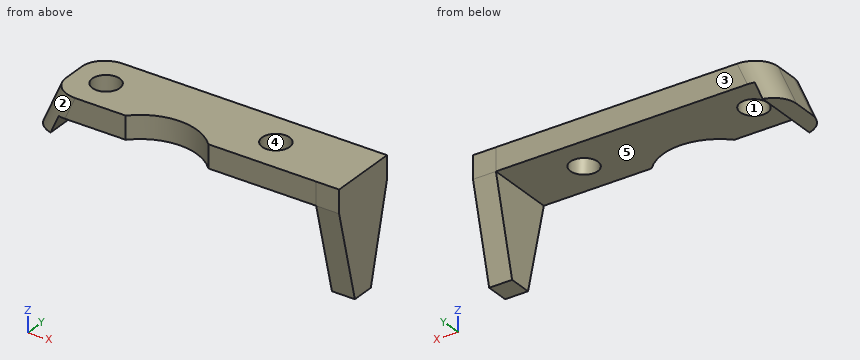
from build123d import *

# Parameters (mm, degrees)
F0_R     = 3
F1_DEPTH = 5
F2_W     = 15.0000307818
F2_H     = 5
F3_DEPTH = 5
F5_DEPTH = 15
F6_R     = 5


with BuildPart() as f1:
    # F0 (on Top) → F1 (new body)
    with BuildSketch(Plane.XY):
        with BuildLine():
            Line((32.4696116149, -7.5), (32.5, 7.5))
            Line((32.5, 7.5), (-25.481024757, 7.5))
            Line((-25.481024757, 7.5), (-25.481024757, 0))
            Line((-25.481024757, 0), (-25.481024757, -7.5))
            Line((-25.481024757, -7.5), (-9, -7.5))
            ThreePointArc((-9, -7.5), (0, -3.6042395476), (9, -7.5))
            Line((9, -7.5), (32.4696116149, -7.5))
        make_face()
        with Locations((-18.481024757, 0)):
            Circle(F0_R, mode=Mode.SUBTRACT)
        with Locations((18.5, 0)):
            Circle(F0_R, mode=Mode.SUBTRACT)
    extrude(amount=F1_DEPTH)

    # F2 (on face) → F3 (join)
    with BuildSketch(Plane(origin=(32.4846724826, -0.0658104491, 0), x_dir=(0.0020258882, 0.9999979479, 0), z_dir=(0.9999979479, -0.0020258882, 0))):
        Polygon((7.565825975, 0), (-7.4342048068, 0), (-2.5, -20), (2.5, -20), align=None)
        with Locations((0.0658105841, 2.5)):
            Rectangle(F2_W, F2_H)
    extrude(amount=F3_DEPTH)

    # F4 (on face) → F5 (join)
    with BuildSketch(Plane.XZ.offset(7.5)):
        Polygon((-29.481024757, -4), (-25.481024757, -4), (-23.7032469792, 0), (-25.481024757, 0), (-25.481024757, 5), align=None)
        Polygon((-25.481024757, 0), (-23.7032469792, 0), (-21.481024757, 5), (-25.481024757, 5), align=None)
    extrude(amount=-F5_DEPTH)

    # F6
    f6_edges = [f1.edges().sort_by_distance(p)[0] for p in [
        (-27.481025, -7.5, 0.5),
        (-27.481025, 7.5, 0.5),
    ]]
    fillet(f6_edges, radius=F6_R)


solid = f1.part
Can you work these out from the model? Positions are in its coordinate system, mm. Face numbers are marked on the shaded views. A direction names the side the tool comes from. Coordinates: 2 decimals unless noted, no trailing zeros. Loops run counter-clockwise (first coordinate to the right, second up) from the corner with the lowest first, then second, coordinate; pieces in that order, holes last. Notation, with made-up numbers: M 26.25,26.5 L 63.25,26.5 A33 cw 63.25,64.5 Z; hole C 1,1.25 d4. An arc over 180 degrees is marked long. Return JSON: item names as keys, results as strings. Group by question number.
Item 1: On a 3-axis mill with a long thin cutter (end or side, diameter ignored), from which of +Z, -Z, +X, -X, +Y, -Y can I reach the whole of each face in a straight line? I mean the marked faces 4 and 5. Say none if no direction works.
Item 2: If I drill on L1, parallel to Y at x = 18.5, z = 3; L2, parallel to Z at x = 21.5, y = 1; L3, parallel to X at y = -3, z = -13.25, over which ranges is the centre line in solid material (lowest first)? Write a range as from..to.
Item 3: Thinking about a two-plate mould opening in X: for the marked faces 1, 2 and 3, which applies, released by +X, released by -X, zero draft, split by the parting line, or undercut?
Item 4: I'm going to push flat-ended pins straight in: pin 1 Ø8 at (x, z) = (15, -2.5) entering from -Y; pin 2 Ø5 at (y, z) = (2, -1.5) entering from +X; pin 3 Ø3.5 at (x, y) = (18.5, 0) entering from -Z; pin 4 Ø2 at (x, y) = (-26.5, -2.5) entering from -Z. Where does each tip first touch, or does it pass through?
Item 5: Imagine slicing it at D-D (z = -13.75). Please give me the cut outline in (x, y).
Item 6: Imagine slicing it at B-B (y = -4.5). Please give me the cut outline in (x, z), and give its area (3 significant figures).
Item 7: Imagine slicing it at A-A (x = 18.5). Please give me the cut outline in (y, z), and give its area (3 significant figures).
Item 8: Imagine slicing it at C-C (y = 0). Please give me the cut outline in (x, z).
Verdict:
{
 "1": {"face 4": "+Z, -Z", "face 5": "-Z, +Y, -Y"},
 "2": {"L1": "y = -7.5..-3, 3..7.5", "L2": "z = 0..5", "L3": "x = 32.48..37.48"},
 "3": {"face 1": "undercut", "face 2": "released by -X", "face 3": "zero draft"},
 "4": {"pin 1": "stops at y = -7.5", "pin 2": "stops at x = 37.49", "pin 3": "passes through", "pin 4": "stops at z = -4"},
 "5": {"outline": "M 32.48,-4.11 L 37.48,-4.12 L 37.49,4.01 L 32.49,4.02 Z"},
 "6": {"outline": "M -29.02,-4 L -25.48,-4 L -23.7,0 L -4.62,0 L -4.62,5 L -25.02,5 Z; M 4.62,0 L 32.48,0 L 32.48,-12.16 L 37.48,-12.2 L 37.48,5 L 4.62,5 Z", "area": "347 mm^2"},
 "7": {"outline": "M -7.5,0 L -3,0 L -3,5 L -7.5,5 Z; M 3,0 L 7.5,0 L 7.5,5 L 3,5 Z", "area": "45.0 mm^2"},
 "8": {"outline": "M -29.48,-4 L -25.48,-4 L -23.7,0 L -21.48,0 L -21.48,5 L -25.48,5 Z; M -15.48,0 L 15.5,0 L 15.5,5 L -15.48,5 Z; M 21.5,0 L 32.48,0 L 32.48,-20 L 37.48,-20 L 37.48,5 L 21.5,5 Z"}
}
